Can you work these out from the model? Positions are in its coordinate system, mm. A direction names the side the tool comes from. Round coordinates to 2 decimals unless told otherwise and drop trailing zeros. Write each loop counter-clockwise with the first axis right and the second up, starting at its lowest first coordinate (ties: lowest second). Pieces come first, ordered by that corner, then holes.
Q1. If we section it at A-A (z = 1.85): Give the number of separate pieces and of enclosed holes in the cut face, plus the area to 3 significant figures.
Q2. For faces 4 (the cylindrical face through (-0.573, -4.363, -1.479)), 5 (the flat face through (1, 3, -3)), 6 (the cylindrical face through (-2.262, -1.734, 1.807)), which set-ups out of +Z, -Z, +X, -X, +Y, -Y let a thin tool reach every point of the face, with its end or its side?
Q3. If we section it at C-C (y = 7.5): Please give me the cut outline in (x, z).
Q4. I'm going to push flat-ended pins straight in: pin 1 Ø2 at (y, z) = (6, 1.5) entering from +X; pin 2 Ø4 at (x, y) = (-0.5, 0) entering from -Z; pin 3 Ø2 at (x, y) = (-3.5, -7.5) entering from +Z; pin 4 Ø4.5 at (x, y) = (0.5, 0) entering from +Z. Where does each tip first touch, or does it pass through?
Q5. Please list where these lines run through material, in increasing order: line 1 along Y through (x, z) = (0, 1.7); line 2 along Y through (x, z) = (0, 1.15); line 3 along Y through (x, z) = (-7.5, 0.8).
Q6. We'd pull the mould along Z, two halves only. Please class faces 1 (the flat face through (4.5, 0.1, 2.3)), 2 (the cylindrical face through (3, 0, -1)), 3 (the flat face through (4.5, -2.2, 0)): +Z half, -Z half, draft (parallel to the pull), parting line (faces both ways), or undercut.
from build123d import *

# Parameters (mm, degrees)
SKETCH1_R                    = 10.4
BOSS_EXTRUDE1_DEPTH          = 2.3
F_96_0_0063_DIAMETER_HOLE1_D = 1.500000048
SKETCH9_R                    = 4.4
SKETCH9_R_2                  = 3
BOSS_EXTRUDE2_DEPTH          = 3
SKETCH10_R                   = 4.35
SKETCH10_R_2                 = 3.4
CUT_EXTRUDE1_DEPTH           = 1
SKETCH11_R                   = 2.85
CUT_EXTRUDE2_DEPTH           = 1
SKETCH12_R                   = 1
CUT_EXTRUDE3_DEPTH           = 4


with BuildPart() as part:
    # Sketch1 → Boss-Extrude1 (new body)
    with BuildSketch(Plane.XY):
        Circle(SKETCH1_R)
    extrude(amount=BOSS_EXTRUDE1_DEPTH)

    # #96 (0.0063) Diameter Hole1 (through all)
    with Locations(Plane.XY.offset(2.3)):
        with Locations((0, 7.5), (-3.5, 7.5), (3.5, 7.5), (-7.5, 0), (-7.584790225, 3.5), (-7.584790225, -3.5)):
            f_96_0_0063_diameter_hole1 = Hole(F_96_0_0063_DIAMETER_HOLE1_D / 2)

    # Mirror1: #96 (0.0063) Diameter Hole1 across plane
    add(f_96_0_0063_diameter_hole1.mirror(Plane.ZX), mode=Mode.SUBTRACT)

    # Mirror2: #96 (0.0063) Diameter Hole1 across plane
    add(f_96_0_0063_diameter_hole1.mirror(Plane(origin=(0, 0, 0), x_dir=(0, 0, 1), z_dir=(1, 0, 0))), mode=Mode.SUBTRACT)

    # Sketch9 → Boss-Extrude2 (add)
    with BuildSketch(Plane(origin=(0, 0, 0), x_dir=(-1, 0, 0), z_dir=(0, 0, -1))):
        with Locations(Location((0, 0, 0), (0, 0, 180))):
            Circle(SKETCH9_R)
        Circle(SKETCH9_R_2, mode=Mode.SUBTRACT)
    extrude(amount=BOSS_EXTRUDE2_DEPTH)

    # Sketch10 → Cut-Extrude1 (cut)
    with BuildSketch(Plane.XY.offset(2.3)):
        Circle(SKETCH10_R)
        Circle(SKETCH10_R_2, mode=Mode.SUBTRACT)
    extrude(amount=-CUT_EXTRUDE1_DEPTH, mode=Mode.SUBTRACT)

    # Sketch11 → Cut-Extrude2 (cut)
    with BuildSketch(Plane.XY.offset(2.3)):
        Circle(SKETCH11_R)
    extrude(amount=-CUT_EXTRUDE2_DEPTH, mode=Mode.SUBTRACT)

    # Sketch12 → Cut-Extrude3 (cut)
    with BuildSketch(Plane.XY.offset(1.3)):
        Circle(SKETCH12_R)
    extrude(amount=-CUT_EXTRUDE3_DEPTH, mode=Mode.SUBTRACT)


solid = part.part
A:
1. separate pieces: 2
1. enclosed holes: 14
1. area: 270 mm2
2. face 4: -Z
2. face 5: -Z, +X, -X, +Y, -Y
2. face 6: +Z
3. outline: (-7.2, 0) - (-4.25, 0) - (-4.25, 2.3) - (-7.2, 2.3) - close; (-2.75, 0) - (-0.75, 0) - (-0.75, 2.3) - (-2.75, 2.3) - close; (0.75, 0) - (2.75, 0) - (2.75, 2.3) - (0.75, 2.3) - close; (4.25, 0) - (7.2, 0) - (7.2, 2.3) - (4.25, 2.3) - close
4. pin 1: stops at x = 9.12
4. pin 2: stops at z = 0
4. pin 3: stops at z = 2.3
4. pin 4: stops at z = 1.3
5. line 1: y = -10.4 to -8.25, -6.75 to -4.35, -3.4 to -2.85, 2.85 to 3.4, 4.35 to 6.75, 8.25 to 10.4
5. line 2: y = -10.4 to -8.25, -6.75 to -1, 1 to 6.75, 8.25 to 10.4
5. line 3: y = -7.2 to -4.25, -2.75 to -0.75, 0.75 to 2.75, 4.25 to 7.2
6. face 1: +Z half
6. face 2: draft
6. face 3: -Z half
